Here's how the part is built. I have some questions about the finished solid (model axes, mm). Face numbers are marked on the shaded views. A direction names the side the tool comes from. Give positions to 0.01 mm unless a question says otherwise; leave off trailing zeros. Order: outer loops, then holes, each group sorted by start corner. A loop starts at its lowest first (then second) coordinate and runs counter-clockwise, first axis right, second up.
from build123d import *

# Parameters (mm, degrees)
BOSS_EXTRUDE3_START     = 44.460213
BOSS_EXTRUDE3_DEPTH     = 19.939
CHAMFER2_SIZE           = 5.08
FILLET2_R               = 3.81
SKETCH4_R               = 2.38125
CUT_EXTRUDE1_DEPTH      = 4.591914717
CUT_EXTRUDE1_DEPTH_BACK = 22.046085283


with BuildPart() as part:
    # Sketch3 → Boss-Extrude3 (new body)
    with BuildSketch(Plane(origin=(0, 0, 0), x_dir=(0, 0, -1), z_dir=(1, 0, 0)).offset(BOSS_EXTRUDE3_START)):
        Polygon((30.787104637, 3.591914717), (30.787104637, -18.352057258), (-10.513295363, -18.352057258), (-10.513295363, 3.591914717), (-18.133295363, 3.591914717), (-18.133295363, -21.046085283), (38.407104637, -21.046085283), (38.407104637, 3.591914717), align=None)
    extrude(amount=BOSS_EXTRUDE3_DEPTH)

    # Chamfer2
    chamfer2_edges = [part.edges().sort_by_distance(p)[0] for p in [
        (54.429713, -18.352057258, 10.513295363),
    ]]
    chamfer(chamfer2_edges, length=CHAMFER2_SIZE)

    # Fillet2
    fillet2_edges = [part.edges().sort_by_distance(p)[0] for p in [
        (54.429713, -18.352057258, -30.787104637),
    ]]
    fillet(fillet2_edges, radius=FILLET2_R)

    # Sketch4 → Cut-Extrude1 (cut, two sides)
    with BuildSketch(Plane(origin=(0, 0, 0), x_dir=(1, 0, 0), z_dir=(0, 1, 0))) as cut_extrude1_sk:
        with Locations((49.444963475, 34.546304637)):
            Circle(SKETCH4_R)
        with Locations((59.414463475, 34.546304637)):
            Circle(SKETCH4_R)
        with Locations((49.444963475, -14.272495363)):
            Circle(SKETCH4_R)
        with Locations((59.414463475, -14.272495363)):
            Circle(SKETCH4_R)
    extrude(amount=CUT_EXTRUDE1_DEPTH, mode=Mode.SUBTRACT)
    extrude(cut_extrude1_sk.sketch, amount=-CUT_EXTRUDE1_DEPTH_BACK, mode=Mode.SUBTRACT)


solid = part.part
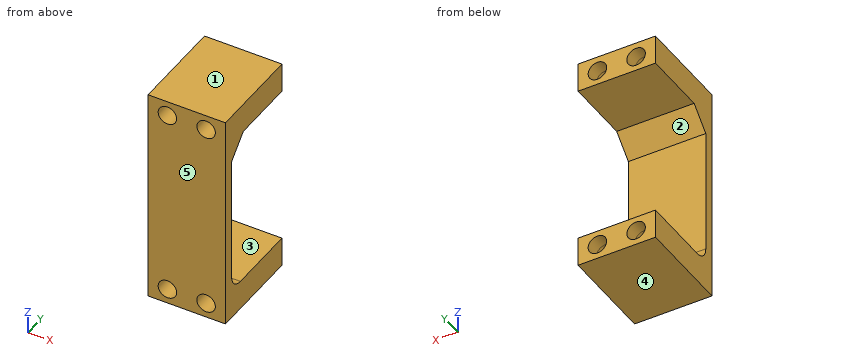
Q1. Thinking about a two-plate mould opening in Z: for the marked faces 3, 4 and 5, which applies, released by +Z, released by -Z, zero draft, split by the parting line, or undercut?
Filled sheet:
face 3: undercut
face 4: released by -Z
face 5: zero draft
Q2. I'm going to push flat-ended pins straight in: P1, Ø10, axis at x = 57.5, z = -3.5, coming from the +Y side; P2, Ø6, axis at x = 48.5, z = 6.5, coming from the +Y side. Where does each tip first touch, or does it pass through?
Filled sheet:
P1: stops at y = -18.35
P2: stops at y = -14.29
Q3. If we section it at A-A on y = -9.75: List the corners of the cut face in (x, z) for me, plus the area to 3 significant figures.
Filled sheet:
outline: (44.46, -38.41) - (64.4, -38.41) - (64.4, -30.79) - (44.46, -30.79) - close; (44.46, 10.51) - (64.4, 10.51) - (64.4, 18.13) - (44.46, 18.13) - close; hole circle Ø4.76 at (49.44, -34.55); hole circle Ø4.76 at (49.44, 14.27); hole circle Ø4.76 at (59.41, -34.55); hole circle Ø4.76 at (59.41, 14.27)
area: 233 mm2
Q4. If we section it at D-D on x = 46.5: List the corners of the cut face in (y, z) for me, plus the area to 3 significant figures.
Filled sheet:
outline: (-21.05, -38.41) - (3.59, -38.41) - (3.59, -30.79) - (-14.54, -30.79) arc R3.81 cw to (-18.35, -26.98) - (-18.35, 5.43) - (-13.27, 10.51) - (3.59, 10.51) - (3.59, 18.13) - (-21.05, 18.13) - close
area: 503 mm2
Q5. I need wall thicknesses on L1, parallel to Z at x = 59.25, y = -9; L2, parallel to Z at x = 53.5, y = 2; L3, parallel to Z at x = 57.75, y = -15. Which ranges of each line are inside material? Lowest first, please.
Filled sheet:
L1: z = -38.41 to -36.92, -32.17 to -30.79, 10.51 to 11.9, 16.65 to 18.13
L2: z = -38.41 to -30.79, 10.51 to 18.13
L3: z = -38.41 to -36.25, -32.84 to -30.76, 8.79 to 12.57, 15.98 to 18.13
Q6. If we section it at B-B on x = 50.75: List the corners of the cut face in (y, z) for me, plus the area to 3 significant figures.
Filled sheet:
outline: (-21.05, -38.41) - (3.59, -38.41) - (3.59, -36.54) - (-21.05, -36.54) - close; (-21.05, -32.55) - (3.59, -32.55) - (3.59, -30.79) - (-14.54, -30.79) arc R3.81 cw to (-18.35, -26.98) - (-18.35, 5.43) - (-13.27, 10.51) - (3.59, 10.51) - (3.59, 12.28) - (-21.05, 12.28) - close; (-21.05, 16.26) - (3.59, 16.26) - (3.59, 18.13) - (-21.05, 18.13) - close
area: 306 mm2
Q7. If we section it at C-C on y = -19.25: List the corners of the cut face in (x, z) for me.
Filled sheet:
outline: (44.46, -38.41) - (64.4, -38.41) - (64.4, 18.13) - (44.46, 18.13) - close; hole circle Ø4.76 at (49.44, -34.55); hole circle Ø4.76 at (49.44, 14.27); hole circle Ø4.76 at (59.41, -34.55); hole circle Ø4.76 at (59.41, 14.27)
Q8. For the marked faces 1 and 2, which set-ups out of +Z, -Z, +X, -X, +Y, -Y let a thin tool reach every point of the face, with its end or its side?
Filled sheet:
face 1: +Z, +X, -X, +Y, -Y
face 2: +X, -X, +Y
